from build123d import *


with BuildPart() as part:
    # Esquisse1 → Révolution1 (revolve)
    with BuildSketch(Plane.XY, mode=Mode.PRIVATE) as r_volution1_sk:
        Polygon((0, -72.517220377), (3.5, -72.517220377), (3.5, -76.017220377), (2.2857838, -76.017220377), (2.2857838, -79.517220377), (3.75, -79.517220377), (3.75, -81.517220377), (6, -81.517220377), (6, -83.017220377), (3.75, -83.017220377), (3.75, -85.517220377), (5, -85.517220377), (5, -95.517220377), (0, -95.517220377), align=None)
    revolve(r_volution1_sk.sketch.rotate(Axis((0, -72.517220377, 0), (0, -1, 0)), 180), axis=Axis((0, -72.517220377, 0), (0, -1, 0)))


solid = part.part
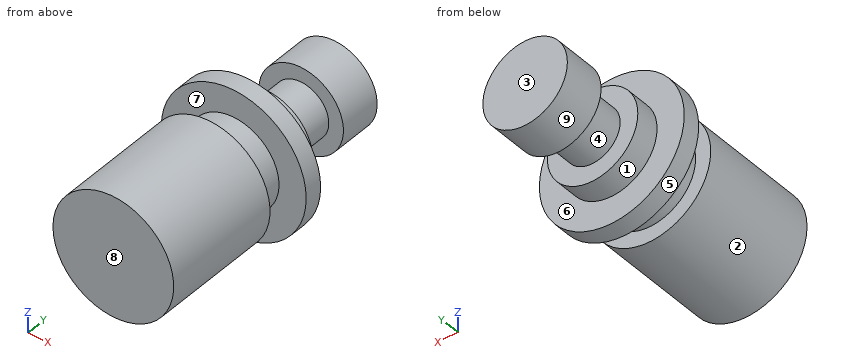
CAD build for the part. Positions are in the model's coordinates, mm. Face numbers are marked on the shaded views. A direction names the side the tool comes from. Give positions to 0.01 mm unless a question says otherwise; leave off trailing zeros. Write each loop counter-clockwise with the first axis right and the second up, starting at its lowest first coordinate (ties: lowest second). Pieces come first, ordered by that corner, then holes. Notation, with made-up numbers: M 41.5,28 L 59.5,28 A25 cw 59.5,43 Z; hole C 23.25,-3.5 d3. An arc over 180 degrees is marked long. Put each result on its own line as item: value. Start each with the question number.
(1) Flat gauge pins, fed straight in: pin 1 Ø4 at (x, y) = (0, -91) entering from -Z; pin 2 Ø2 at (x, y) = (3, -88) entering from +Z; pin 3 Ø1 at (y, z) = (-86.5, -4.5) entering from +X. Where does each tip first touch, or does it go through?
(2) Band-saw the part on B-B, the plane x = 0. Write the cut outline in (y, z).
(3) Band-saw the part on D-D, the plane x = -4.75. Write the cut outline in (y, z).
(4) Which spindle directions (+Z, -Z, +X, -X, +Y, -Y) get a long thin tool onto all of the face, cutting with end or side? Do the marked faces 1, 2, 3, 4 and 5. Say none if no direction does.
(5) Band-saw the part on C-C, the plane z = 0. Write the cut outline in (x, y), and give its area (3 significant figures).
(6) Probe L1, parallel to Y at x = 1.25, z = 4.75; L2, parallel to Y at x = -2.25, z = 5.25; L3, parallel to Y at x = -2.75, z = -0.5. List the from-to ranges inside material, lowest first.
(7) Mould opens along Y. For the marked faces 6, 7, 8 and 9 say: +Y half, -Y half, draft (parallel to the pull), parting line (faces both ways), or undercut.
(8) Band-saw the part on A-A, the plane z = -4. Write the cut outline in (x, y), and give its area (3 significant figures).
Response values:
1. pin 1: stops at z = -5
1. pin 2: stops at z = 4.58
1. pin 3: stops at x = 3
2. outline: M -95.52,-5 L -85.52,-5 L -85.52,-3.75 L -83.02,-3.75 L -83.02,-6 L -81.52,-6 L -81.52,-3.75 L -79.52,-3.75 L -79.52,-2.29 L -76.02,-2.29 L -76.02,-3.5 L -72.52,-3.5 L -72.52,3.5 L -76.02,3.5 L -76.02,2.29 L -79.52,2.29 L -79.52,3.75 L -81.52,3.75 L -81.52,6 L -83.02,6 L -83.02,3.75 L -85.52,3.75 L -85.52,5 L -95.52,5 Z
3. outline: M -95.52,-1.56 L -85.52,-1.56 L -85.52,1.56 L -95.52,1.56 Z; M -83.02,-3.67 L -81.52,-3.67 L -81.52,3.67 L -83.02,3.67 Z
4. face 1: +Y
4. face 2: -Y
4. face 3: +Z, -Z, +X, -X, +Y
4. face 4: none
4. face 5: +Y, -Y
5. outline: M -6,-83.02 L -3.75,-83.02 L -3.75,-85.52 L -5,-85.52 L -5,-95.52 L 5,-95.52 L 5,-85.52 L 3.75,-85.52 L 3.75,-83.02 L 6,-83.02 L 6,-81.52 L 3.75,-81.52 L 3.75,-79.52 L 2.29,-79.52 L 2.29,-76.02 L 3.5,-76.02 L 3.5,-72.52 L -3.5,-72.52 L -3.5,-76.02 L -2.29,-76.02 L -2.29,-79.52 L -3.75,-79.52 L -3.75,-81.52 L -6,-81.52 Z
5. area: 192 mm2
6. L1: y = -95.52 to -85.52, -83.02 to -81.52
6. L2: y = -83.02 to -81.52
6. L3: y = -95.52 to -79.52, -76.02 to -72.52
7. face 6: +Y half
7. face 7: undercut
7. face 8: -Y half
7. face 9: draft
8. outline: M -4.47,-83.02 L 4.47,-83.02 L 4.47,-81.52 L -4.47,-81.52 Z; M -3,-95.52 L 3,-95.52 L 3,-85.52 L -3,-85.52 Z
8. area: 73.4 mm2
